Build history of the part. All positions in model axes, mm. A direction names the side the tool comes from. Give positions to 0.01 mm unless a question says otherwise; leave off trailing zeros. Order: outer loops, then holes, each group sorted by start corner. A loop starts at its lowest first (then second) coordinate and runs counter-clockwise, first axis right, second up. Notation, with made-up numbers: (85.5, -37) - (125.5, -37) arc R29 ccw to (125.5, -6) - close; hole circle Ø6 at (86.25, 78). An arc over 180 degrees is marked (long way). Use a Markdown table: item, result.
from build123d import *

# Parameters (mm, degrees)
EXTRUDE_1_DEPTH     = 6
SKETCH_5_R          = 2
SKETCH_5_R_2        = 1.5
CUT_EXTRUDE_3_DEPTH = 53.172568548
FILLET_1_R          = 4


with BuildPart() as part:
    # d → 凸台-拉伸1 (new body)
    # profile 1 of 2: a face of its own
    with BuildSketch(Plane.XY):
        Polygon((-5.930243874, -4), (7.416343955, 29.033964073), (29.583656045, 29.033964073), (42.930243874, -4), align=None)
        Polygon((0, 0), (37, 0), (26.885621978, 25.033964073), (10.114378022, 25.033964073), align=None, mode=Mode.SUBTRACT)
    # profile 2 of 2: a face of its own
    with BuildSketch(Plane.XY):
        Polygon((0, 0), (10.114378022, 25.033964073), (26.885621978, 25.033964073), (37, 0), align=None)
        Polygon((5.930243874, 4), (31.069756126, 4), (24.18758791, 21.033964073), (12.81241209, 21.033964073), align=None, mode=Mode.SUBTRACT)
    extrude(amount=EXTRUDE_1_DEPTH)

    # 草图5 → 切除-拉伸3 (cut, through all)
    with BuildSketch(Plane.XY.offset(6)):
        Circle(SKETCH_5_R)
        with Locations((37, 0)):
            Circle(SKETCH_5_R)
        with Locations((26.885621978, 25.033964073)):
            Circle(SKETCH_5_R_2)
        with Locations((10.114378022, 25.033964073)):
            Circle(SKETCH_5_R_2)
    extrude(amount=-CUT_EXTRUDE_3_DEPTH, mode=Mode.SUBTRACT)

    # 圆角1
    fillet_1_edges = [part.edges().sort_by_distance(p)[0] for p in [
        (31.069756126, 4, 3),
        (24.18758791, 21.033964073, 3),
        (12.81241209, 21.033964073, 3),
        (5.930243874, 4, 3),
        (7.416343955, 29.033964073, 3),
        (29.583656045, 29.033964073, 3),
        (42.930243874, -4, 3),
        (-5.930243874, -4, 3),
    ]]
    fillet(fillet_1_edges, radius=FILLET_1_R)


solid = part.part
1) Tool access for faces 4 (the cylindrical face through (-3.346, -2.191, 3.042)), 5 (the flat face through (10.002, 14.079, 2.958)): list every direction of +Z, -Z, +X, -X, +Y, -Y with a clear straight run to the whole face (end or side of a thin tool).
Computed:
| item | result |
|---|---|
| face 4 | +Z, -Z, -X |
| face 5 | +Z, -Z |
2) Two-plate mould, pull along Y, no slides. Class faces 1 (the flat face through (19, 2, 6)), 2 (the flat face through (27.05, 13.95, 2.96)), 3 (the flat face through (1.278, 13.84, 2.958)): +Y half, -Y half, draft (parallel to the pull), parting line (faces both ways), or undercut.
Computed:
| item | result |
|---|---|
| face 1 | draft |
| face 2 | undercut |
| face 3 | +Y half |
3) Slice it at C-C (z = 4.6). Write the cut outline in (x, y), and give its area (3 significant figures).
Computed:
| item | result |
|---|---|
| outline | (-3.71, 1.5) arc R4 ccw to (0, -4) - (37, -4) arc R4 ccw to (40.71, 1.5) - (30.59, 26.53) arc R4 ccw to (26.89, 29.03) - (10.11, 29.03) arc R4 ccw to (6.41, 26.53) - close; hole circle Ø4 at (0, 0); hole (8.15, 9.5) arc R4 ccw to (11.86, 4) - (25.14, 4) arc R4 ccw to (28.85, 9.5) - (25.2, 18.53) arc R4 ccw to (21.49, 21.03) - (15.51, 21.03) arc R4 ccw to (11.8, 18.53) - close; hole circle Ø3 at (10.11, 25.03); hole circle Ø3 at (26.89, 25.03); hole circle Ø4 at (37, 0) |
| area | 823 mm² |
4) Slice it at A-A (x = 19). Write the cut outline in (y, z), and give its area (3 significant figures).
Computed:
| item | result |
|---|---|
| outline | (-4, 0) - (4, 0) - (4, 6) - (-4, 6) - close; (21.03, 0) - (29.03, 0) - (29.03, 6) - (21.03, 6) - close |
| area | 96.0 mm² |
5) Pin check, flat tips, straight feed: P1, Ø1.5, axis at x = 18, y = -0.5, coming from the -Z side; P2, Ø1.8, axis at x = 26.89, y = 25.03, coming from the +Z side. Stop position of each tip, or through.
Computed:
| item | result |
|---|---|
| P1 | stops at z = 0 |
| P2 | passes through |
6) Slice it at D-D (y = 17). Write the cut outline in (x, z).
Computed:
| item | result |
|---|---|
| outline | (2.55, 0) - (11.18, 0) - (11.18, 6) - (2.55, 6) - close; (25.82, 0) - (34.45, 0) - (34.45, 6) - (25.82, 6) - close |
7) Wall check: line 1 (X direction, y = 26, z = 0.4); line 2 (X direction, y = 16, z = 2.35); line 3 (Y direction, x = 9, z = 2.85). Give the ranges that are in metal, low to high. Write a range as from..to.
Computed:
| item | result |
|---|---|
| line 1 | x = 6.19..8.97, 11.26..25.74, 28.03..30.81 |
| line 2 | x = 2.15..10.78, 26.22..34.85 |
| line 3 | y = -4..5.2, 11.6..24.03, 26.04..28.88 |
8) Slice it at B-B (y = 0). Write the cut outline in (x, z).
Computed:
| item | result |
|---|---|
| outline | (-4, 0) - (-2, 0) - (-2, 6) - (-4, 6) - close; (2, 0) - (35, 0) - (35, 6) - (2, 6) - close; (39, 0) - (41, 0) - (41, 6) - (39, 6) - close |
